Part model, mm, in its own coordinate system. A direction names the side the tool comes from. Coordinates: 2 decimals unless noted, no trailing zeros. Order: outer loops, then holes, each group sorted by start corner. A loop starts at its lowest first (then second) coordinate and runs counter-clockwise, first axis right, second up. Notation, with made-up numbers: (62, 7) - (99, 7) arc R19 cw to (99, 39) - close; hole circle Ø6 at (-1.75, -31.75). An arc over 180 degrees is marked (long way). Use a Markdown table: item, result. Add a question column.
1) Two-plate mould, pull along Z, no slides. Class faces 4 (the face through (1, 100, -111)), 5 (the face through (-3, -1, -125)), 6 (the face through (-235, -1, 2)): +Z half, -Z half, draft (parallel to the pull), parting line (faces both ways), or undercut.
2) Drop flat-ended pins along their axis: P1, Ø5.5, axis at x = 100, z = -100.5, coming from the +Y side; P2, Ø10, axis at x = -11, z = -54.5, coming from the +Y side. Give the stop position or say it passes through.
3) Wall check: L1, parallel to X at y = 81.75, z = -100; L2, parallel to Z at x = 162.5, y = 78; L3, parallel to X at y = -4.5, z = -1. Give the ranges that are in metal, low to high. Write a range as [from, to].
4) Saw through at C-C on x = 213. List the corners of the cut face in (y, z), then the cut area to 4 significant figures.
5) Saw through at D-D on y = 41. List the corners of the cut face in (x, z).
6) Tool access for faces 1 (the face through (-3, -80, -2)), 2 (the face through (242.6, 1.4, 96.72)), 3 (the face through (-2, 88, -110)): list every direction of +Z, -Z, +X, -X, +Y, -Y with a clear straight run to the whole face (end or side of a thin tool).
7) Saw through at A-A on y = 0. List the corners of the cut face in (x, z).
8) Saw through at B-B on z = 65. List the corners of the cut face in (x, y), then the cut area to 3 significant figures.
```python
from build123d import *

# Parameters (mm, degrees)
SKETCH1_W                = 250
SKETCH1_H                = 200
BOSS_EXTRUDE1_DEPTH      = 250
SKETCH7_W                = 470
SKETCH7_H                = 230
CUT_EXTRUDE4_DEPTH       = 80
SKETCH5_R                = 31.75
F_63_5MM_DIA_SERVO_DEPTH = 20
MIRROR13_COPY_1_SKETCH_R = 31.75
MIRROR13_COPY_1_DEPTH    = 20
SKETCH10_W               = 350
SKETCH10_H               = 220
CUT_EXTRUDE5_DEPTH       = 20
SKETCH15_W               = 500
SKETCH15_H               = 250
BOSS_EXTRUDE2_DEPTH      = 10
SKETCH18_W               = 300
SKETCH18_H               = 220
CUT_EXTRUDE11_DEPTH      = 10
SKETCH19_R               = 3.5
CUT_EXTRUDE12_DEPTH      = 10
MIRROR15_COPY_1_SKETCH_R = 3.5
MIRROR15_COPY_1_DEPTH    = 10
SKETCH20_R               = 3.5
CUT_EXTRUDE13_DEPTH      = 10
MIRROR17_COPY_1_SKETCH_R = 3.5
MIRROR17_COPY_1_DEPTH    = 10


with BuildPart() as part:
    # Sketch1 → Boss-Extrude1 (new, symmetric)
    with BuildSketch(Plane(origin=(0, 0, 0), x_dir=(0, 0, -1), z_dir=(1, 0, 0))):
        Rectangle(SKETCH1_W, SKETCH1_H)
    extrude(amount=BOSS_EXTRUDE1_DEPTH, both=True)

    # Sketch7 → Cut-Extrude4 (cut, symmetric)
    with BuildSketch(Plane(origin=(0, 0, 0), x_dir=(1, 0, 0), z_dir=(0, 1, 0))):
        Rectangle(SKETCH7_W, SKETCH7_H)
    extrude(amount=CUT_EXTRUDE4_DEPTH, both=True, mode=Mode.SUBTRACT)

    # Sketch5 → 63.5mm_dia_servo (cut)
    with BuildSketch(Plane(origin=(250, 0, 0), x_dir=(0, 0, -1), z_dir=(1, 0, 0))):
        with Locations((-65, 0)):
            Circle(SKETCH5_R)
    f_63_5mm_dia_servo = extrude(amount=-F_63_5MM_DIA_SERVO_DEPTH, mode=Mode.SUBTRACT)

    # Mirror12: 63.5mm_dia_servo across plane
    add(f_63_5mm_dia_servo.mirror(Plane.XY), mode=Mode.SUBTRACT)

    # Mirror13: 63.5mm_dia_servo across plane
    add(f_63_5mm_dia_servo.mirror(Plane(origin=(0, 0, 0), x_dir=(0, 0, 1), z_dir=(1, 0, 0))), mode=Mode.SUBTRACT)

    # Mirror13 copy 1 sketch → Mirror13 copy 1 (cut)
    with BuildSketch(Plane.ZY.offset(250)):
        with Locations((-65, 0)):
            Circle(MIRROR13_COPY_1_SKETCH_R)
    extrude(amount=-MIRROR13_COPY_1_DEPTH, mode=Mode.SUBTRACT)

    # Sketch10 → Cut-Extrude5 (cut)
    with BuildSketch(Plane(origin=(0, 100, 0), x_dir=(1, 0, 0), z_dir=(0, 1, 0))):
        Rectangle(SKETCH10_W, SKETCH10_H)
    extrude(amount=-CUT_EXTRUDE5_DEPTH, mode=Mode.SUBTRACT)

    # Sketch15 → Boss-Extrude2 (add)
    with BuildSketch(Plane(origin=(0, 75, 0), x_dir=(1, 0, 0), z_dir=(0, 1, 0))):
        Rectangle(SKETCH15_W, SKETCH15_H)
    extrude(amount=BOSS_EXTRUDE2_DEPTH)

    # Sketch18 → Cut-Extrude11 (cut)
    with BuildSketch(Plane(origin=(0, 85, 0), x_dir=(1, 0, 0), z_dir=(0, 1, 0))):
        Rectangle(SKETCH18_W, SKETCH18_H)
    extrude(amount=-CUT_EXTRUDE11_DEPTH, mode=Mode.SUBTRACT)

    # Sketch19 → Cut-Extrude12 (cut)
    with BuildSketch(Plane(origin=(0, 85, 0), x_dir=(1, 0, 0), z_dir=(0, 1, 0))):
        with Locations(Location((-162.5, 100, 0), (0, 0, 270))):
            Circle(SKETCH19_R)
    cut_extrude12 = extrude(amount=-CUT_EXTRUDE12_DEPTH, mode=Mode.SUBTRACT)

    # Mirror14: Cut-Extrude12 across plane
    add(cut_extrude12.mirror(Plane.XY), mode=Mode.SUBTRACT)

    # Mirror15: Cut-Extrude12 across plane
    add(cut_extrude12.mirror(Plane(origin=(0, 0, 0), x_dir=(0, 0, 1), z_dir=(1, 0, 0))), mode=Mode.SUBTRACT)

    # Mirror15 copy 1 sketch → Mirror15 copy 1 (cut)
    with BuildSketch(Plane(origin=(0, 85, 0), x_dir=(-1, 0, 0), z_dir=(0, 1, 0))):
        with Locations(Location((-162.5, 100, 0), (0, 0, 270))):
            Circle(MIRROR15_COPY_1_SKETCH_R)
    extrude(amount=-MIRROR15_COPY_1_DEPTH, mode=Mode.SUBTRACT)

    # Sketch20 → Cut-Extrude13 (cut)
    with BuildSketch(Plane(origin=(0, -80, 0), x_dir=(1, 0, 0), z_dir=(0, 1, 0))):
        with Locations(Location((-100, 100, 0), (0, 0, 270))):
            Circle(SKETCH20_R)
    cut_extrude13 = extrude(amount=-CUT_EXTRUDE13_DEPTH, mode=Mode.SUBTRACT)

    # Mirror16: Cut-Extrude13 across plane
    add(cut_extrude13.mirror(Plane.XY), mode=Mode.SUBTRACT)

    # Mirror17: Cut-Extrude13 across plane
    add(cut_extrude13.mirror(Plane(origin=(0, 0, 0), x_dir=(0, 0, 1), z_dir=(1, 0, 0))), mode=Mode.SUBTRACT)

    # Mirror17 copy 1 sketch → Mirror17 copy 1 (cut)
    with BuildSketch(Plane(origin=(0, -80, 0), x_dir=(-1, 0, 0), z_dir=(0, 1, 0))):
        with Locations(Location((-100, 100, 0), (0, 0, 270))):
            Circle(MIRROR17_COPY_1_SKETCH_R)
    extrude(amount=-MIRROR17_COPY_1_DEPTH, mode=Mode.SUBTRACT)


solid = part.part
```
Results are:
| question | item | result |
|---|---|---|
| 1 | face 4 | draft |
| 1 | face 5 | -Z half |
| 1 | face 6 | undercut |
| 2 | P1 | y = -90 |
| 2 | P2 | y = -80 |
| 3 | L1 | [-250, -166], [-159, -150], [150, 159], [166, 250] |
| 3 | L2 | [-125, -103.5], [-96.5, 96.5], [103.5, 125] |
| 3 | L3 | [-250, -235], [235, 250] |
| 4 | outline | (-100, -125) - (100, -125) - (100, 125) - (-100, 125) - close; hole (-80, -115) - (75, -115) - (75, 115) - (-80, 115) - close |
| 4 | area | 14,350 mm2 |
| 5 | outline | (-250, -125) - (250, -125) - (250, 125) - (-250, 125) - close; hole (-235, -115) - (235, -115) - (235, 115) - (-235, 115) - close |
| 6 | face 1 | none |
| 6 | face 2 | +X, -X |
| 6 | face 3 | +Y |
| 7 | outline | (-250, -125) - (250, -125) - (250, -96.75) - (235, -96.75) - (235, -115) - (-235, -115) - (-235, -96.75) - (-250, -96.75) - close; (-250, -33.25) - (-235, -33.25) - (-235, 33.25) - (-250, 33.25) - close; (-250, 96.75) - (-235, 96.75) - (-235, 115) - (235, 115) - (235, 96.75) - (250, 96.75) - (250, 125) - (-250, 125) - close; (235, -33.25) - (250, -33.25) - (250, 33.25) - (235, 33.25) - close |
| 8 | outline | (-250, -100) - (250, -100) - (250, -31.75) - (235, -31.75) - (235, -80) - (-235, -80) - (-235, -31.75) - (-250, -31.75) - close; (-250, 31.75) - (-235, 31.75) - (-235, 75) - (-150, 75) - (-150, 85) - (-175, 85) - (-175, 100) - (-250, 100) - close; (150, 75) - (235, 75) - (235, 31.75) - (250, 31.75) - (250, 100) - (175, 100) - (175, 85) - (150, 85) - close |
| 8 | area | 17,000 mm2 |
